Autodesk Inventor part; units mm, degrees
ref_plane "YZ Plane" through (0, 0, 0) normal (1, 0, 0) x (0, 1, 0)
ref_plane "XZ Plane" through (0, 0, 0) normal (0, 1, 0) x (-1, 0, 0)
ref_plane "XY Plane" through (0, 0, 0) normal (0, 0, 1) x (1, 0, 0)
sketch "Sketch1" plane through (0, 0, 0) normal (0, 1, 0) x (-1, 0, 0)
  circle A0 centre (0, 0) radius 2.921
  dimension "d0" = 5.842
extrude "Extrusion1" add sketch "Sketch1" along normal blind 6.35
sketch "Sketch2" plane through (0, 0, 0) normal (0, -1, 0) x (1, 0, 0)
  circle A0 centre (0, 0) radius 2.921
  line L0 (-4.1275, -0.4128) -> (4.1275, -0.4128)
  line L1 (4.1275, -0.4128) -> (4.1275, 0.4128)
  line L2 (4.1275, 0.4128) -> (-4.1275, 0.4128)
  line L3 (-4.1275, 0.4128) -> (-4.1275, -0.4128)
  line L4 (-4.1275, -0.4128) -> (4.1275, 0.4128) construction
  line L5 (4.1275, -0.4128) -> (-4.1275, 0.4128) construction
  line L6 (3.7809, 1.7063) -> (3.3681, 2.4212)
  line L7 (-3.3681, -2.4212) -> (3.7809, 1.7063)
  line L8 (3.3681, 2.4212) -> (-3.7809, -1.7063)
  line L9 (-3.7809, -1.7063) -> (-3.3681, -2.4212)
  line L10 (2.4212, 3.3681) -> (1.7063, 3.7809)
  line L11 (-1.7063, -3.7809) -> (2.4212, 3.3681)
  line L12 (1.7063, 3.7809) -> (-2.4212, -3.3681)
  line L13 (-2.4212, -3.3681) -> (-1.7063, -3.7809)
  line L14 (0.4128, 4.1275) -> (-0.4127, 4.1275)
  line L15 (0.4127, -4.1275) -> (0.4128, 4.1275)
  line L16 (-0.4127, 4.1275) -> (-0.4128, -4.1275)
  line L17 (-0.4128, -4.1275) -> (0.4127, -4.1275)
  line L18 (-1.7063, 3.7809) -> (-2.4212, 3.3681)
  line L19 (2.4212, -3.3681) -> (-1.7063, 3.7809)
  line L20 (-2.4212, 3.3681) -> (1.7063, -3.7809)
  line L21 (1.7063, -3.7809) -> (2.4212, -3.3681)
  line L22 (-3.3681, 2.4212) -> (-3.7809, 1.7063)
  line L23 (3.7809, -1.7063) -> (-3.3681, 2.4212)
  line L24 (-3.7809, 1.7063) -> (3.3681, -2.4212)
  line L25 (3.3681, -2.4212) -> (3.7809, -1.7063)
  line L26 (-4.1275, 0.4128) -> (-4.1275, -0.4127)
  line L27 (4.1275, 0.4127) -> (-4.1275, 0.4128)
  line L28 (-4.1275, -0.4127) -> (4.1275, -0.4128)
  line L29 (4.1275, -0.4128) -> (4.1275, 0.4127)
  line L30 (-3.7809, -1.7063) -> (-3.3681, -2.4212)
  line L31 (3.3681, 2.4212) -> (-3.7809, -1.7063)
  line L32 (-3.3681, -2.4212) -> (3.7809, 1.7063)
  line L33 (3.7809, 1.7063) -> (3.3681, 2.4212)
  line L34 (-2.4212, -3.3681) -> (-1.7063, -3.7809)
  line L35 (1.7063, 3.7809) -> (-2.4212, -3.3681)
  line L36 (-1.7063, -3.7809) -> (2.4212, 3.3681)
  line L37 (2.4212, 3.3681) -> (1.7063, 3.7809)
  line L38 (-0.4128, -4.1275) -> (0.4127, -4.1275)
  line L39 (-0.4127, 4.1275) -> (-0.4128, -4.1275)
  line L40 (0.4127, -4.1275) -> (0.4128, 4.1275)
  line L41 (0.4128, 4.1275) -> (-0.4127, 4.1275)
  line L42 (1.7063, -3.7809) -> (2.4212, -3.3681)
  line L43 (-2.4212, 3.3681) -> (1.7063, -3.7809)
  line L44 (2.4212, -3.3681) -> (-1.7063, 3.7809)
  line L45 (-1.7063, 3.7809) -> (-2.4212, 3.3681)
  line L46 (3.3681, -2.4212) -> (3.7809, -1.7063)
  line L47 (-3.7809, 1.7063) -> (3.3681, -2.4212)
  line L48 (3.7809, -1.7063) -> (-3.3681, 2.4212)
  line L49 (-3.3681, 2.4212) -> (-3.7809, 1.7063)
  circle A1 centre (0, 0) radius 3.175
  circle A2 centre (0, 0) radius 3.175
  point P0 (2.9327, -1.2166)
  point P1 (3.1481, -0.4127)
  point P2 (3.1481, 0.4128)
  point P3 (2.9327, 1.2166)
  point P4 (2.5199, 1.9315)
  point P5 (1.9315, 2.5199)
  point P6 (1.2166, 2.9327)
  point P7 (0.4128, 3.1481)
  point P8 (-0.4128, 3.1481)
  point P9 (-1.2166, 2.9327)
  point P10 (-1.9315, 2.5199)
  point P11 (-2.5199, 1.9315)
  point P12 (-2.9327, 1.2166)
  point P13 (-3.1481, 0.4127)
  point P14 (-3.1481, -0.4128)
  point P15 (-2.9327, -1.2166)
  point P16 (-2.5199, -1.9315)
  point P17 (-1.9315, -2.5199)
  point P18 (-1.2166, -2.9327)
  point P19 (-0.4128, -3.1481)
  point P20 (0.4127, -3.1481)
  point P21 (1.2166, -2.9327)
  point P22 (1.9315, -2.5199)
  point P23 (2.5199, -1.9315)
  dimension "d5" = 8.255
  dimension "d6" = 0.8255
  dimension "d7" = 360
extrude "Extrusion2" add sketch "Sketch2" along normal blind 3.175
fillet "Fillet1" radius 0.3175 2 edges at (2.4212, -1.5875, 3.3681) (1.7063, -1.5875, 3.7809)
pattern_circular "Circular Pattern1" count 12 over 360 about axis through (0, 0, 0) along (0, 1, 0) of "Fillet1", "Extrusion1"
fillet "Fillet2" radius 0.3175 1 edges at (2.921, 6.35, 0)
sketch "Sketch3" plane through (0, -3.175, 0) normal (0, -1, 0) x (1, 0, 0)
  line L0 (-1.5875, -1.5875) -> (1.5875, -1.5875)
  line L1 (1.5875, -1.5875) -> (1.5875, 1.5875)
  line L2 (1.5875, 1.5875) -> (-1.5875, 1.5875)
  line L3 (-1.5875, 1.5875) -> (-1.5875, -1.5875)
  line L4 (-1.5875, -1.5875) -> (1.5875, 1.5875) construction
  line L5 (1.5875, -1.5875) -> (-1.5875, 1.5875) construction
  point P0 (0, 0)
  dimension "d15" = 3.175
  dimension "d16" = 3.175
extrude "Extrusion3" cut sketch "Sketch3" against normal blind 3.175
sketch "Sketch4" plane through (0, 6.35, 0) normal (0, 1, 0) x (1, 0, 0)
  circle A0 centre (0, 0) radius 2.921
  circle A1 centre (0, 0) radius 2.921
  circle A2 centre (0, 0) radius 2.794
  dimension "d19" = 5.588
extrude "Extrusion4" cut sketch "Sketch4" against normal blind 6.35
properties part number "Gear1"
Build history of the part. All positions in model axes, mm. A direction names the side the tool comes from. Round coordinates to 2 decimals unless told otherwise and drop trailing zeros. Use CSV: the item, a comma, the result in double quotes.
(1) Wall check: line 1 (X direction, y = -1, z = 3.5); line 2 (Z direction, x = 3.25, y = -1); line 3 (Z direction, x = 2, y = -0.25). Give the ranges that are in metal, low to high.
Response:
line 1,"-2.19 to -1.54, -0.41 to 0.41, 1.54 to 2.19"
line 2,"-2.3 to -1.4, -0.41 to 0.41, 1.4 to 2.3"
line 3,"-3.61 to -2.64, -2.47 to 2.47, 2.64 to 3.61"
(2) 3-axis set-ups, long thin cutter, end or side, ignore diameter. For faces 5 (the cylindrical face through (-0.816, -1.565, -3.068)), 6 (the cylindrical face through (-0.827, -1.565, 3.065)), 7 (the flat face through (0, -2, 1.588)): which of +Z, -Z, +X, -X, +Y, -Y reach the whole face in a straight line?
Response:
face 5,"-Z, +Y, -Y"
face 6,"+Z, +Y, -Y"
face 7,"-Y"
(3) Pin check, flat tips, straight feed: P1, Ø0.7, axis at x = -3.5, y = -1.5, coming from the +Z side (3 decimals); P2, Ø1, axis at y = 3, z = 0, coming from the -X side; P3, Ø1.6, axis at x = 0.5, z = 0.5, coming from the -Y side. Stop position of each tip, or through.
Response:
P1,"z = 2.305"
P2,"x = -2.79"
P3,"y = 0"
(4) Mould opens along Z. For faces 1 (the cylindrical face through (0.827, -1.565, -3.065)), 2 (the cylindrical face through (0.816, -1.565, 3.068)), 3 (the flat face through (0, -2, -1.588)), 4 (the flat face through (0, 0, 0)) say: pulls with the +Z half, pulls with the -Z half, needs draft (parallel to the pull), parting line crosses it, or undercut.
Response:
face 1,"pulls with the -Z half"
face 2,"pulls with the +Z half"
face 3,"undercut"
face 4,"undercut"
